```python
from build123d import *

# Parameters (mm, degrees)
BOSS_EXTRUDE1_DEPTH           = 70
SKETCH8_R                     = 4.5
CUT_EXTRUDE4_DEPTH            = 53.5
SKETCH10_R                    = 7.05
CUT_EXTRUDE5_DEPTH            = 4
FILLET13_R                    = 1
M8_CLEARANCE_HOLE1_AT_2_COUNT = 2
M8_CLEARANCE_HOLE1_AT_2_PITCH = 24.109474775


with BuildPart() as part:
    # Sketch1 → Boss-Extrude1 (new body)
    with BuildSketch(Plane(origin=(0, 0, 0), x_dir=(1, 0, 0), z_dir=(0, 1, 0))):
        Polygon((-26.25, -26.25), (26.25, -26.25), (26.25, 19.75), (20.25, 19.75), (20.25, -20.25), (-20.25, -20.25), (-20.25, 19.75), (-26.25, 19.75), align=None)
    extrude(amount=BOSS_EXTRUDE1_DEPTH)

    # Sketch8 → Cut-Extrude4 (cut, through all)
    with BuildSketch(Plane(origin=(26.25, 0, 0), x_dir=(0, 0, -1), z_dir=(1, 0, 0))):
        with Locations((-0.25, 55)):
            Circle(SKETCH8_R)
    extrude(amount=-CUT_EXTRUDE4_DEPTH, mode=Mode.SUBTRACT)

    # Sketch10 → Cut-Extrude5 (cut)
    with BuildSketch(Plane.ZY.offset(26.25)):
        with Locations((0.25, 55)):
            Circle(SKETCH10_R)
    cut_extrude5 = extrude(amount=-CUT_EXTRUDE5_DEPTH, mode=Mode.SUBTRACT)

    # Mirror1: Cut-Extrude5 across plane
    add(cut_extrude5.mirror(Plane(origin=(0, 0, 0), x_dir=(0, 0, 1), z_dir=(1, 0, 0))), mode=Mode.SUBTRACT)

    # Fillet13
    fillet13_edges = [part.edges().sort_by_distance(p)[0] for p in [
        (26.25, 0, 3.25),
        (0, 0, 26.25),
        (0, 70, 20.25),
        (-26.25, 0, 3.25),
        (-23.25, 0, -19.75),
        (-20.25, 0, 0.25),
        (0, 0, 20.25),
        (20.25, 0, 0.25),
        (-20.25, 70, 0.25),
        (20.25, 35, -19.75),
        (26.25, 35, -19.75),
        (26.25, 35, 26.25),
        (-26.25, 35, 26.25),
        (-26.25, 35, -19.75),
        (-20.25, 35, -19.75),
        (-23.25, 70, -19.75),
        (-26.25, 70, 3.25),
        (0, 70, 26.25),
        (26.25, 70, 3.25),
        (23.25, 70, -19.75),
        (20.25, 70, 0.25),
        (23.25, 0, -19.75),
    ]]
    fillet(fillet13_edges, radius=FILLET13_R)

    # Sketch18 → M8 Clearance Hole1 (revolve, cut)
    with BuildSketch(Plane(origin=(-20.25, 35.786178525, 0.25), x_dir=(0, 0, -1), z_dir=(0, 1, 0))):
        Polygon((0, 0), (0, 15.703872786), (4.5, 13), (4.5, 0.025), (4.525, 0), align=None)
    m8_clearance_hole1 = revolve(axis=Axis((-13.9, 35.786178525, 0.25), (-1, 0, 0)), mode=Mode.SUBTRACT)

    # M8 Clearance Hole1 at 2: M8 Clearance Hole1 ×2
    with Locations(*[(0, -i * M8_CLEARANCE_HOLE1_AT_2_PITCH, 0) for i in range(1, M8_CLEARANCE_HOLE1_AT_2_COUNT)]):
        add(m8_clearance_hole1, mode=Mode.SUBTRACT)

    # Mirror2: M8 Clearance Hole1 across plane
    add(m8_clearance_hole1.mirror(Plane(origin=(0, 0, 0), x_dir=(0, 0, 1), z_dir=(1, 0, 0))), mode=Mode.SUBTRACT)

    # Mirror2 copy 1 sketch → Mirror2 copy 1 (revolve, cut)
    with BuildSketch(Plane(origin=(20.25, 11.676703751, 0.25), x_dir=(0, 0, -1), z_dir=(0, 1, 0))):
        Polygon((0, 0), (0, -15.703872786), (4.5, -13), (4.5, -0.025), (4.525, 0), align=None)
    revolve(axis=Axis((13.9, 11.676703751, 0.25), (-1, 0, 0)), mode=Mode.SUBTRACT)


solid = part.part
```
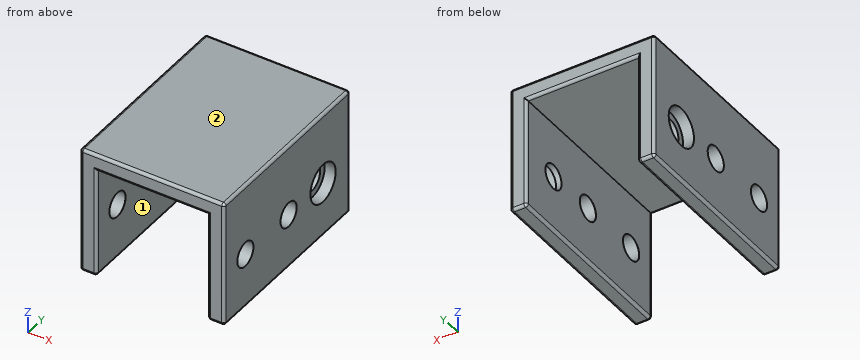
Check sheet for the modelled part. Datum: model origin and axes. Units: mm. Face numbers are marked on the shaded views. A direction names the side the tool comes from. Give positions to 0.01 mm unless a question says otherwise; leave off trailing zeros. Order: outer loops, then holes, each group sorted by start corner. A loop starts at its lowest first (then second) coordinate and runs counter-clockwise, first axis right, second up. Notation, with made-up numbers: M 56,11.5 L 111,11.5 A8 ccw 111,22.5 Z; hole C 21.25,43 d1. An arc over 180 degrees is marked long. Answer in a Markdown table with one row per item.
1) Access from +Z, -Z, +X, -X, +Y, -Y to the whole of each face (thin tool, end or side, straight path). Record for the marked faces 1 and 2.
Filled sheet:
| item | result |
|---|---|
| face 1 | -Z, +Y, -Y |
| face 2 | +Z, +X, -X, +Y, -Y |
2) Cross-section at B-B, the plane y = 55. Count the separate pieces of the cut face and the enclosed holes in it, plus the area to 3 significant figures.
Filled sheet:
| item | result |
|---|---|
| separate pieces | 3 |
| enclosed holes | 0 |
| area | 645 mm2 |
3) Gauge pin test, flat ends, axial feed: P1, Ø10.5, axis at y = 55, z = 0.25, coming from the -X side; P2, Ø10.5, axis at y = 55, z = 0.25, coming from the +X side. Record the tip position at first contact, or that the pin passes through.
Filled sheet:
| item | result |
|---|---|
| P1 | stops at x = -22.25 |
| P2 | stops at x = 22.25 |
4) Cross-section at D-D, the plane y = 43. Enter the section's corners in (x, z).
Filled sheet:
| item | result |
|---|---|
| outline | M -26.25,-18.75 A1 ccw -25.25,-19.75 L -21.25,-19.75 A1 ccw -20.25,-18.75 L -20.25,20.25 L 20.25,20.25 L 20.25,-18.75 A1 ccw 21.25,-19.75 L 25.25,-19.75 A1 ccw 26.25,-18.75 L 26.25,25.25 A1 ccw 25.25,26.25 L -25.25,26.25 A1 ccw -26.25,25.25 Z |
5) Cross-section at C-C, the plane x = 15. Enter the section's corners in (y, z), plus the area to 3 significant figures.
Filled sheet:
| item | result |
|---|---|
| outline | M 0,21.25 A1 ccw 1,20.25 L 69,20.25 A1 ccw 70,21.25 L 70,25.25 A1 ccw 69,26.25 L 1,26.25 A1 ccw 0,25.25 Z |
| area | 419 mm2 |
6) Cross-section at A-A, the plane z = 15.5. Enter the section's corners in (x, y), plus the area to 3 significant figures.
Filled sheet:
| item | result |
|---|---|
| outline | M -26.25,1 A1 ccw -25.25,0 L -21.25,0 A1 ccw -20.25,1 L -20.25,69 A1 ccw -21.25,70 L -25.25,70 A1 ccw -26.25,69 Z; M 20.25,1 A1 ccw 21.25,0 L 25.25,0 A1 ccw 26.25,1 L 26.25,69 A1 ccw 25.25,70 L 21.25,70 A1 ccw 20.25,69 Z |
| area | 838 mm2 |
7) Thickness scan on L1, parallel to Y at x = -24.3, z = 0.25; L2, parallel to X at y = 35, z = 15; L3, parallel to Y at x = -21, z = 0. Record the ranges inside material, lowest first. Write a range as [from, to].
Filled sheet:
| item | result |
|---|---|
| L1 | y = [0, 7.18], [16.18, 31.29], [40.29, 47.95], [62.05, 70] |
| L2 | x = [-26.25, -20.25], [20.25, 26.25] |
| L3 | y = [0.03, 7.18], [16.17, 31.29], [40.28, 50.51], [59.49, 69.97] |
